Autodesk Inventor part; units mm, degrees
ref_plane "YZ Plane" through (0, 0, 0) normal (1, 0, 0) x (0, 1, 0)
ref_plane "XZ Plane" through (0, 0, 0) normal (0, 1, 0) x (-1, 0, 0)
ref_plane "XY Plane" through (0, 0, 0) normal (0, 0, 1) x (1, 0, 0)
sketch "Sketch1" plane through (0, 0, 0) normal (0, 0, 1) x (1, 0, 0)
  line L0 (-11.9516, 53) -> (17.0484, 53)
  line L1 (23.0484, 47) -> (23.0484, 43)
  line L2 (3.0484, 23) -> (-1.9516, 23)
  line L3 (-11.9516, 33) -> (-11.9516, 53)
  arc A0 (23.0484, 47) -> (17.0484, 53) centre (17.0484, 47) ccw
  arc A1 (3.0484, 23) -> (23.0484, 43) centre (3.0484, 43) ccw
  arc A2 (-11.9516, 33) -> (-1.9516, 23) centre (-1.9516, 33) ccw
  point P0 (0, 0)
  point P1 (23.0484, 23)
  point P2 (-11.9516, 23)
  dimension "d0" = 6
  dimension "d1" = 30
  dimension "d2" = 35
  dimension "d3" = 20
  dimension "d4" = 10
extrude "Extrusion1" add sketch "Sketch1" along normal blind 5
sketch "Sketch3" plane through (0, 0, 0) normal (0, 0, -1) x (-1, 0, 0)
  line L0 (-17.0484, 53) -> (11.9516, 53)
  line L1 (11.9516, 53) -> (11.9516, 33)
  line L2 (11.9516, 53) -> (11.9516, 33)
  arc A0 (1.9516, 23) -> (11.9516, 33) centre (1.9516, 33) ccw
  line L3 (1.9516, 23) -> (-3.0484, 23)
  line L4 (1.9516, 23) -> (-3.0484, 23)
  line L5 (-23.0484, 43) -> (-23.0484, 47)
  line L6 (-23.0484, 43) -> (-23.0484, 47)
  arc A1 (-17.0484, 53) -> (-23.0484, 47) centre (-17.0484, 47) ccw
  line L7 (-17.0484, 53) -> (11.9516, 53)
  arc A2 (1.9516, 23) -> (11.9516, 33) centre (1.9516, 33) ccw
  arc A3 (-23.0484, 43) -> (-3.0484, 23) centre (-3.0484, 43) ccw
  arc A4 (-17.0484, 53) -> (-23.0484, 47) centre (-17.0484, 47) ccw
  line L8 (11.4516, 52.5) -> (11.4516, 33.5)
  line L9 (-2.5484, 23.5) -> (1.4516, 23.5)
  line L10 (-22.5484, 46.5) -> (-22.5484, 43.5)
  line L11 (-16.5484, 52.5) -> (11.4516, 52.5)
  arc A5 (-16.5484, 52.5) -> (-22.5484, 46.5) centre (-16.5484, 46.5) ccw
  arc A6 (1.4516, 23.5) -> (11.4516, 33.5) centre (1.4516, 33.5) ccw
  arc A7 (-22.5484, 43.5) -> (-2.5484, 23.5) centre (-2.5484, 43.5) ccw
  point P0 (0, 0)
  dimension "d14" = 10
  dimension "d15" = 20
  dimension "d16" = 6
  dimension "d17" = 0.5
  dimension "d18" = 0.5
  dimension "d19" = 0.5
  dimension "d20" = 0.5
  dimension "d21" = 6
  dimension "d22" = 10
  dimension "d23" = 20
extrude "Extrusion2" add sketch "Sketch3" along normal blind 1.5
sketch "Sketch4" plane through (0, 0, 5) normal (0, 0, 1) x (1, 0, 0)
  line L0 (-1.9516, 23) -> (3.0484, 23)
  arc A0 (3.0484, 23) -> (23.0484, 43) centre (3.0484, 43) ccw
  line L1 (23.0484, 43) -> (23.0484, 47)
  arc A1 (23.0484, 47) -> (17.0484, 53) centre (17.0484, 47) ccw
  line L2 (17.0484, 53) -> (-11.9516, 53)
  line L3 (-11.9516, 53) -> (-11.9516, 33)
  arc A2 (-11.9516, 33) -> (-1.9516, 23) centre (-1.9516, 33) ccw
  line L4 (-9.9516, 50) -> (10.0484, 50)
  line L5 (10.0484, 50) -> (10.0484, 49)
  line L6 (10.0484, 49) -> (-9.9516, 49)
  line L7 (-9.9516, 49) -> (-9.9516, 50)
  point P0 (0, 0)
  dimension "d26" = 1
  dimension "d27" = 3
  dimension "d28" = 2
  dimension "d29" = 20
extrude "Extrusion3" add sketch "Sketch4" along normal blind 10 contours L4 L5 L6 L7
properties part number "McCrea_oko_walle"
Can you work these out from the model? Positions are in its coordinate system, mm. A direction names the side the tool comes from. Coordinates: 2 decimals unless noted, no trailing zeros. Loops run counter-clockwise (first coordinate to the right, second up) from the corner with the lowest first, then second, coordinate; pieces in that order, holes last. Notation, with made-up numbers: (31, 30) -> (60, 30) arc R25 cw to (60, 62) -> close; hole circle Ø1 at (44.25, 16). An arc over 180 degrees is marked (long way). Answer as a JSON object with one key per item and string values.
1) For faces 1 (the face through (20.837, 50.696, -0.74)), 2 (the face through (10.048, 49.5, 9.9)), 3 (the face through (0, 50, 10)), which set-ups out of +Z, -Z, +X, -X, +Y, -Y let a thin tool reach every point of the face, with its end or its side?
Results:
{"face 1": "-Z", "face 2": "+Z, +X, +Y, -Y", "face 3": "+Z, +X, -X, +Y"}
2) Imagine slicing it at B-B (z = 2). Please give me the cut outline in (x, y).
Results:
{"outline": "(-11.95, 33) arc R10 ccw to (-1.95, 23) -> (3.05, 23) arc R20 ccw to (23.05, 43) -> (23.05, 47) arc R6 ccw to (17.05, 53) -> (-11.95, 53) -> close"}
3) Imagine slicing it at C-C (x = -1). Please give me the cut outline in (y, z).
Results:
{"outline": "(23, -1.5) -> (23.5, -1.5) -> (23.5, 0) -> (52.5, 0) -> (52.5, -1.5) -> (53, -1.5) -> (53, 5) -> (50, 5) -> (50, 15) -> (49, 15) -> (49, 5) -> (23, 5) -> close"}
4) For P1, Ø8, axis at x = 2.5, z = 11, coming from the -Y side; P2, Ø0.8, axis at x = 4, z = -1, coming from the -Y side; P3, Ø6, axis at x = 18, y = 36, coming from the +Z side, each with a flat end and sliding along its axis, tell me the tip position at first contact or that it passes through.
Results:
{"P1": "stops at y = 49", "P2": "stops at y = 23.01", "P3": "stops at z = 5"}
5) Imagine slicing it at A-A (y = 44). Please give me the cut outline in (x, z), then the cut area to 4 significant figures.
Results:
{"outline": "(-11.95, -1.5) -> (-11.45, -1.5) -> (-11.45, 0) -> (22.55, 0) -> (22.55, -1.5) -> (23.05, -1.5) -> (23.05, 5) -> (-11.95, 5) -> close", "area": "176.5 mm^2"}
6) Thinking about a two-plate mould opening in Y: for faces 4 (the face through (21.244, 51.289, 1.704)), 5 (the face through (-9.952, 49.5, 9.9)), 6 (the face through (1, 23.5, -1)), which applies, pulls with the +Y half, pulls with the -Y half, needs draft (parallel to the pull), parting line crosses it, or undercut?
Results:
{"face 4": "pulls with the +Y half", "face 5": "needs draft", "face 6": "undercut"}
7) If I drill on line 1 (Z direction, x = 11, y = 31); line 2 (X direction, y = 27.25, z = -0.5); line 3 (Z direction, x = -7, y = 49.75), over which ranges is the centre line in solid material (lowest first)?
Results:
{"line 1": "z = 0 to 5", "line 2": "x = -10.13 to -9.26, 14.21 to 15.37", "line 3": "z = 0 to 15"}
8) Imagine slicing it at D-D (x = -4.5). Please give me the cut outline in (y, z).
Results:
{"outline": "(23.33, -1.5) -> (23.98, -1.5) -> (23.98, 0) -> (52.5, 0) -> (52.5, -1.5) -> (53, -1.5) -> (53, 5) -> (50, 5) -> (50, 15) -> (49, 15) -> (49, 5) -> (23.33, 5) -> close"}
